Here's the drawing with two shaded views (mm, measured from the low corner). I have some questions. Coordinates: 2 decimals unless noted, no trailing zeros. Loops run counter-clockwise (first coordinate to the right, second up) from the corner with the lowest first, then second, coordinate; pieces in that order, holes last. Notation, with made-up numbers: (34.5, -32) -> (80.5, -32) arc R12 ccw to (80.5, -14) -> close; hole circle Ø6 at (19, -15.5). An arc over 180 degrees is marked (long way). Answer as a JSON object with one key per item and string values. Group by question number.
Q1. I'm going to push a flat-ended pin straight in: pin 1 (1 mm diameter, centred on x = 15, y = 25.4, fed in from -Z). Where does the tip first touch, or does it pass through?
Q2. I want a section at A-A on y = 17.6. Write out the boundary of the cut face in (x, z).
Q3. I want a section at B-B on z = 1.3. Count the separate pieces of the cut face and the enclosed holes in it, then the cut area to 3 significant figures.
Q4. I need wall thicknesses on line 1 (X direction, y = 22.8, z = 1). Which ranges of the line are inside material? Lowest first, please.
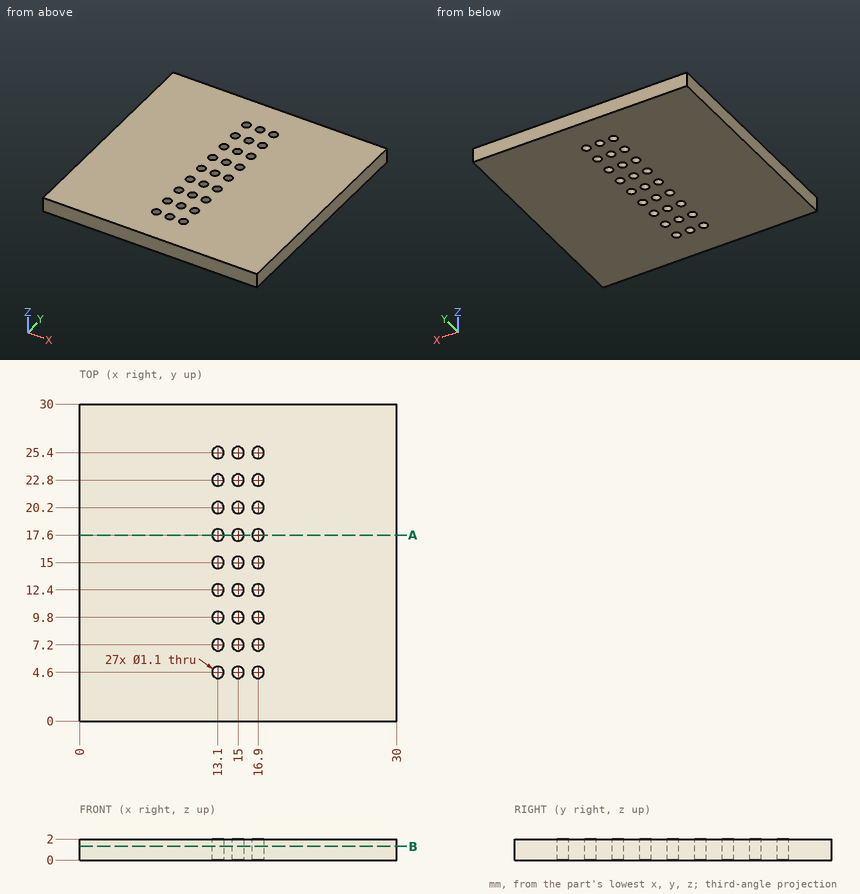
Result set:
{
 "1": {"pin 1": "passes through"},
 "2": {"outline": "(0, 0) -> (12.55, 0) -> (12.55, 2) -> (0, 2) -> close; (13.65, 0) -> (14.45, 0) -> (14.45, 2) -> (13.65, 2) -> close; (15.55, 0) -> (16.35, 0) -> (16.35, 2) -> (15.55, 2) -> close; (17.45, 0) -> (30, 0) -> (30, 2) -> (17.45, 2) -> close"},
 "3": {"separate pieces": "1", "enclosed holes": "27", "area": "874 mm²"},
 "4": {"line 1": "x = 0 to 12.55, 13.65 to 14.45, 15.55 to 16.35, 17.45 to 30"}
}
